For this review, take the finished solid that the model builds, in its own axes (mm). Coordinates: 2 decimals unless noted, no trailing zeros. Loops run counter-clockwise (first coordinate to the right, second up) from the corner with the lowest first, then second, coordinate; pieces in that order, holes last. Notation, with made-up numbers: M 39.5,43 L 91.5,43 A10 ccw 91.5,54 Z; hole C -30,27.25 d2. An arc over 180 degrees is marked long. Write item = value, one per line.
from build123d import *

# Parameters (mm, degrees)
SKETCH_1_W      = 68
SKETCH_1_H      = 80
SKETCH_1_R      = 4.1
SKETCH_1_R_2    = 2.1
EXTRUDE_1_DEPTH = 3
CHAMFER_1_SIZE  = 25
CHAMFER_2_SIZE  = 4
CHAMFER_3_SIZE  = 2


with BuildPart() as part:
    # 草图1 → 凸台-拉伸1 (new, symmetric)
    with BuildSketch(Plane.XY):
        with Locations((9, 10)):
            Rectangle(SKETCH_1_W, SKETCH_1_H)
        Circle(SKETCH_1_R, mode=Mode.SUBTRACT)
        with Locations((35, 20)):
            Circle(SKETCH_1_R_2, mode=Mode.SUBTRACT)
        with Locations((35, -20)):
            Circle(SKETCH_1_R_2, mode=Mode.SUBTRACT)
        with Locations((-15, 40)):
            Circle(SKETCH_1_R_2, mode=Mode.SUBTRACT)
        with Locations((15, 40)):
            Circle(SKETCH_1_R_2, mode=Mode.SUBTRACT)
    extrude(amount=EXTRUDE_1_DEPTH, both=True)

    # 倒角1
    chamfer_1_edges = [part.edges().sort_by_distance(p)[0] for p in [
        (43, 50, 0),
    ]]
    chamfer(chamfer_1_edges, length=CHAMFER_1_SIZE)

    # 倒角2
    chamfer_2_edges = [part.edges().sort_by_distance(p)[0] for p in [
        (-4.1, 0, 3),
        (-25, 50, 0),
        (43, -30, 0),
        (-25, -30, 0),
    ]]
    chamfer(chamfer_2_edges, length=CHAMFER_2_SIZE)

    # 倒角3
    chamfer_3_edges = [part.edges().sort_by_distance(p)[0] for p in [
        (32.9, 20, 3),
        (32.9, -20, 3),
        (-17.1, 40, 3),
        (12.9, 40, 3),
    ]]
    chamfer(chamfer_3_edges, length=CHAMFER_3_SIZE)


solid = part.part
Q1. Add section A-A (x = 15). Write out the cut boundary in (y, z).
Solved:
outline = M -30,-3 L 37.9,-3 L 37.9,1 L 35.9,3 L -30,3 Z; M 42.1,-3 L 50,-3 L 50,3 L 44.1,3 L 42.1,1 Z
Q2. Draft analysis for pull direction X (two halves, no side actions). For faces 1 (the face through (41, -28, 0)), 2 (the face through (-23, 48, 0)), 3 (the face through (4.1, 1.3, -0.8)), 4 (the face through (14.54, 37.95, -1.03)), state which applies: +X half, -X half, draft (parallel to the pull), parting line (faces both ways), or undercut.
Solved:
face_1 = +X half
face_2 = -X half
face_3 = undercut
face_4 = undercut
Q3. Add section C-C (y = 40). Write out the cut boundary in (x, z), and give its area (3 significant figures).
Solved:
outline = M -25,-3 L -17.1,-3 L -17.1,1 L -19.1,3 L -25,3 Z; M -12.9,-3 L 12.9,-3 L 12.9,1 L 10.9,3 L -10.9,3 L -12.9,1 Z; M 17.1,-3 L 28,-3 L 28,3 L 19.1,3 L 17.1,1 Z
area = 260 mm²
Q4. For line 1 along Y through (x, z) = (35, -1.1); line 2 along Y through (x, z) = (0, -2.1); line 3 along X through (y, z) = (29, 2), list the stretches that pass through material, from the lowest coordinate up.
Solved:
line_1 = -30 to -22.1, -17.9 to 17.9, 22.1 to 33
line_2 = -30 to -4.1, 4.1 to 50
line_3 = -25 to 39
Q5. Add section B-B (y = 20). Write out the cut boundary in (x, z), and give its area (3 significant figures).
Solved:
outline = M -25,-3 L 32.9,-3 L 32.9,1 L 30.9,3 L -25,3 Z; M 37.1,-3 L 43,-3 L 43,3 L 39.1,3 L 37.1,1 Z
area = 379 mm²
Q6. For pin 1 Ø2.5 at (x, y) = (35, -20) entering from -Z; pin 2 Ø6.5 at (x, y) = (-15, 40) entering from +Z, all flat-tipped, find the tip position at first contact; note any pin that passes through.
Solved:
pin_1 = through
pin_2 = 2.15
Q7. Add section D-D (z = -2). Write out the cut boundary in (x, y), and give its area (3 significant figures).
Solved:
outline = M -25,-26 L -21,-30 L 39,-30 L 43,-26 L 43,25 L 18,50 L -21,50 L -25,46 Z; hole C -15,40 d4.2; hole C 0,0 d8.2; hole C 15,40 d4.2; hole C 35,-20 d4.2; hole C 35,20 d4.2
area = 5,000 mm²
